Read the model definition and answer for the solid it produces. Units are mm, in the model's axes. Give positions to 0.01 mm unless a question says otherwise; leave off trailing zeros. Write each loop counter-clockwise with the first axis right and the second up, starting at its lowest first coordinate (ties: lowest second). Pieces come first, ordered by that corner, then holes. Notation, with made-up numbers: (61, 83.25) -> (104, 83.25) arc R24 cw to (104, 112.25) -> close; hole circle Ø2 at (16.5, -11). An arc over 180 degrees is marked (long way). Answer as CSV lines item,"result". Start each with the question number.
1. The part is cut by section A-A, the plane x = 278.13. Determine the outline of the cut face in (y, z) (3 decimals), and give its area (3 significant figures).
2. The part is cut by section B-B, the plane y = 0. Determine the outline of the cut face in (x, z) (3 decimals), and give its area (3 significant figures).
3. For a pull along Y with two mould halves and no side action, classify faces 1 (the cylindrical face through (294.836, 0.738, -0.044)), 2 (the flat face through (150, -12.7, 0)), 3 (the flat face through (150, 12.7, 0)) as pulls with the +Y half, pulls with the -Y half, needs draft (parallel to the pull), parting line crosses it, or undercut.
4. Find the intervals of material crossed by line 1 (Y direction, x = 278.13, z = -0.5); line 2 (X direction, y = 0.75, z = 1.75); line 3 (X direction, y = 1.5, z = -0.25), in increasing order.
5. Given pin 1 (6.5 mm diameter, centred on x = 278.13, y = 0, fed in from +Z) (3 decimals), flat-ended and moving along its own axis, determine where the tip first touches the part or whether it passes through.
from build123d import *

# Parameters (mm, degrees)
SKETCH1_W                        = 304.8
SKETCH1_H                        = 25.4
BOSS_EXTRUDE1_DEPTH              = 3.175
F_10_0_1935_DIAMETER_HOLE1_D     = 4.9149
F_10_0_1935_DIAMETER_HOLE1_DEPTH = 11.938
F_10_0_1935_DIAMETER_HOLE1_TIP   = 1.476584928


with BuildPart() as part:
    # Sketch1 → Boss-Extrude1 (new body, symmetric)
    with BuildSketch(Plane.XY):
        with Locations((152.4, 0)):
            Rectangle(SKETCH1_W, SKETCH1_H)
    extrude(amount=BOSS_EXTRUDE1_DEPTH, both=True)

    # #10 (0.1935) Diameter Hole1
    with Locations(Plane.XY.offset(3.175)):
        with Locations((7.62, 0), (26.67, 0), (278.13, 0), (297.18, 0)):
            Hole(F_10_0_1935_DIAMETER_HOLE1_D / 2, depth=F_10_0_1935_DIAMETER_HOLE1_DEPTH)
            with Locations((0, 0, -(F_10_0_1935_DIAMETER_HOLE1_DEPTH + F_10_0_1935_DIAMETER_HOLE1_TIP / 2))):  # 118° drill point
                Cone(0, F_10_0_1935_DIAMETER_HOLE1_D / 2, F_10_0_1935_DIAMETER_HOLE1_TIP, mode=Mode.SUBTRACT)


solid = part.part
Results found:
1,outline,"(-12.7, -3.175) -> (-2.457, -3.175) -> (-2.457, 3.175) -> (-12.7, 3.175) -> close; (2.457, -3.175) -> (12.7, -3.175) -> (12.7, 3.175) -> (2.457, 3.175) -> close"
1,area,"130 mm²"
2,outline,"(0, -3.175) -> (5.163, -3.175) -> (5.163, 3.175) -> (0, 3.175) -> close; (10.077, -3.175) -> (24.213, -3.175) -> (24.213, 3.175) -> (10.077, 3.175) -> close; (29.127, -3.175) -> (275.673, -3.175) -> (275.673, 3.175) -> (29.127, 3.175) -> close; (280.587, -3.175) -> (294.723, -3.175) -> (294.723, 3.175) -> (280.587, 3.175) -> close; (299.637, -3.175) -> (304.8, -3.175) -> (304.8, 3.175) -> (299.637, 3.175) -> close"
2,area,"1,810 mm²"
3,face 1,"undercut"
3,face 2,"pulls with the -Y half"
3,face 3,"pulls with the +Y half"
4,line 1,"y = -12.7 to -2.46, 2.46 to 12.7"
4,line 2,"x = 0 to 5.28, 9.96 to 24.33, 29.01 to 275.79, 280.47 to 294.84, 299.52 to 304.8"
4,line 3,"x = 0 to 5.67, 9.57 to 24.72, 28.62 to 276.18, 280.08 to 295.23, 299.13 to 304.8"
5,pin 1,"stops at z = 3.175"
